Design review of the part shown in the three views and the two pictorial views. Dimensions are in mm from the part's minimum x, y and z. A direction names the side the tool comes from. Round coordinates to 2 decimals unless told otherwise and drop trailing zeros. Loops run counter-clockwise (first coordinate to the right, second up) from the corner with the lowest first, then second, coordinate; pieces in that order, holes last. Notation, with made-up numbers: M 72.5,10 L 103.5,10 A20 cw 103.5,15 Z; hole C -18.5,2 d3. An arc over 180 degrees is marked long. One line per question, with ' | ' between items. Start each with the question number.
1) We need section C-C (x = 5). Give the boundary of the cut face in (y, z).
2) For the marked faces 4, 5 and 6, list the 3-axis set-ups (+Z, -Z, +X, -X, +Y, -Y) from which the entire face can be reached by the end or side of a thin tool; tool diameter is ignored.
3) We need section D-D (z = 2.25). Give the boundary of the cut face in (x, y), and give its area (3 significant figures).
4) Mouldability with a two-part tool opening along Y and no side actions: class the marked faces 1, 2 and 3 as pulls with the +Y half, pulls with the -Y half, needs draft (parallel to the pull), parting line crosses it, or undercut.
5) For probe 1 along Y at (x, z) = (11, 3.25); probe 2 along X at (y, z) = (11, 2.25), list the stretches that pass through material, from the lowest coordinate up. Write a range as from..to.
6) We need section B-B (z = 7.5). Give the boundary of the cut face in (x, y), and give its area (3 significant figures).
7) For pin 1 Ø1.5 at (x, y) = (29, 1) entering from +Z; pin 2 Ø4 at (x, z) = (32.5, 10.5) entering from +Y; pin 3 Ø7.5 at (x, y) = (77, 13) entering from +Z, all flat-tipped, find the tip position at first contact; note any pin that passes through.
8) We need section A-A (y = 21). Give the boundary of the cut face in (x, z), and give its area (3 significant figures).
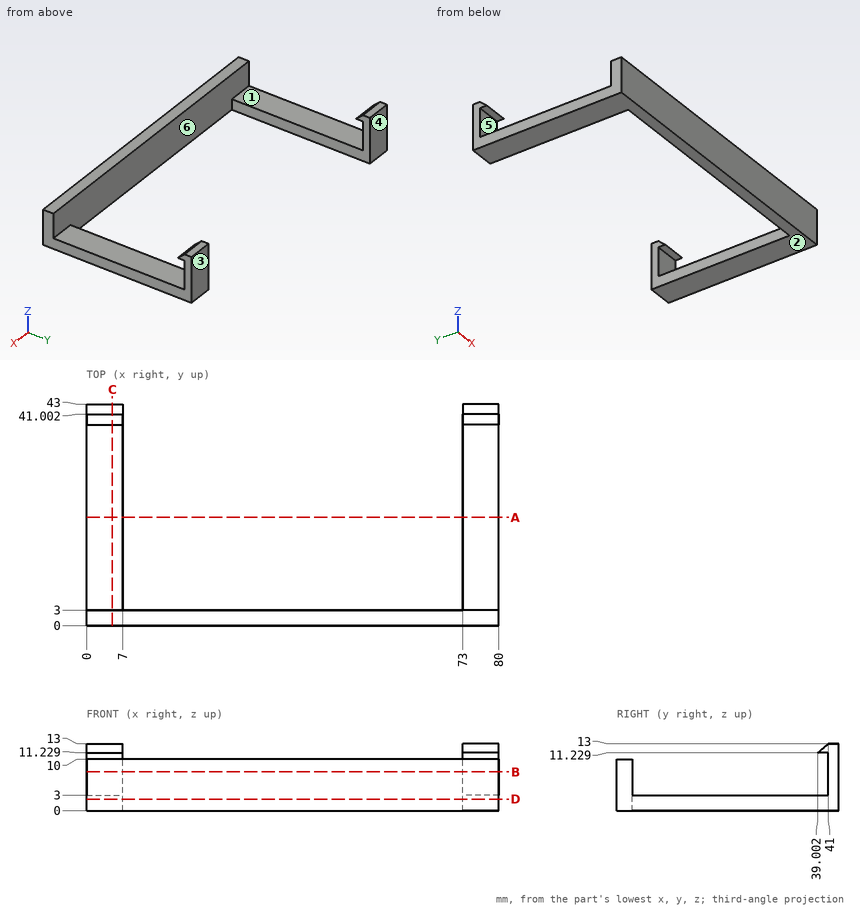
Answers below:
1) outline: M 0,0 L 43,0 L 43,13 L 41,13 L 39,11.23 L 41,11.23 L 41,3 L 3,3 L 3,10 L 0,10 Z
2) face 4: +Z, -Z, +X, -X, +Y | face 5: +X, -X | face 6: +Z
3) outline: M 0,0 L 80,0 L 80,43 L 73,43 L 73,3 L 7,3 L 7,43 L 0,43 Z | area: 800 mm^2
4) face 1: undercut | face 2: needs draft | face 3: pulls with the +Y half
5) probe 1: 0..3 | probe 2: 0..7, 73..80
6) outline: M 0,0 L 80,0 L 80,3 L 0,3 Z; M 0,41 L 7,41 L 7,43 L 0,43 Z; M 73,41 L 80,41 L 80,43 L 73,43 Z | area: 268 mm^2
7) pin 1: z = 10 | pin 2: y = 3 | pin 3: z = 3
8) outline: M 0,0 L 7,0 L 7,3 L 0,3 Z; M 73,0 L 80,0 L 80,3 L 73,3 Z | area: 42.0 mm^2
